from build123d import *

# Parameters (mm, degrees)
F0_W     = 12.5
F0_H     = 3
F0_W_2   = 6
F0_H_2   = 2
F0_W_3   = 44
F0_H_3   = 6
F0_H_4   = 1.2
F1_DEPTH = 580
F3_DEPTH = 50
F5_DEPTH = 50


with BuildPart() as f1:
    # F0 (on Right) → F1 (new body)
    with BuildSketch(Plane.YZ):
        with Locations((6.25, 1.5)):
            Rectangle(F0_W, F0_H)
        with Locations((15.5, 1.5)):
            Rectangle(F0_W_2, F0_H)
        with Locations((6.25, 4)):
            Rectangle(F0_W, F0_H_2)
        with Locations((40.5, 1.5)):
            Rectangle(F0_W_3, F0_H)
        with Locations((15.5, 4)):
            Rectangle(F0_W_2, F0_H_2)
        Polygon((18.5, 5), (18.5, 3), (62.5, 3), (52.9347826087, 5), align=None)
        with Locations((15.5, 8)):
            Rectangle(F0_W_2, F0_H_3)
        Polygon((18.5, 11), (18.5, 5), (52.9347826087, 5), (24.2391304348, 11), align=None)
        with Locations((15.5, 11.6)):
            Rectangle(F0_W_2, F0_H_4)
        Polygon((18.5, 12.2), (18.5, 11), (24.2391304348, 11), align=None)
    extrude(amount=F1_DEPTH)

    # F2 (on Top) → F3 (cut, symmetric)
    with BuildSketch(Plane.XY):
        Polygon((0, 62.5), (0, 0), (62.5, 0), align=None)
    extrude(amount=F3_DEPTH, both=True, mode=Mode.SUBTRACT)

    # F4 (on Top) → F5 (cut, symmetric)
    with BuildSketch(Plane.XY):
        Polygon((580, 62.5), (517.5, 0), (580, 0), align=None)
    extrude(amount=F5_DEPTH, both=True, mode=Mode.SUBTRACT)


solid = f1.part
Work out the finished part from the listing and answer in its coordinate system (mm). A direction names the side the tool comes from. Coordinates: 2 decimals unless noted, no trailing zeros. Order: outer loops, then holes, each group sorted by start corner. A loop starts at its lowest first (then second) coordinate and runs counter-clockwise, first axis right, second up. Notation, with made-up numbers: (-25, 6.25) - (22, 6.25) arc R22 cw to (22, 39.25) - close; hole circle Ø3 at (24, 73.25). An arc over 180 degrees is marked (long way). Put each result on its own line as item: value. Start each with the question number.
1) Find section B-B (y = 7). Give the vertices of the cut face in (x, z), plus the area to 4 significant figures.
2) Find section C-C (y = 45). Give the vertices of the cut face in (x, z).
3) Find the intervals of material crossed by line 1 (Z direction, x = 237, y = 6.5); line 2 (Z direction, x = 95, y = 39); line 3 (X direction, y = 38, z = 3.25), in increasing order. Write a range as from..to.
4) Flat-ended cylindrical pins translate along their axes: pin 1 (5 mm diameter, centred on y = 25.5, z = 8.5, fed in from -X); pin 2 (4 mm diameter, centred on x = 107, y = 54.5, fed in from +Z); pin 3 (10 mm diameter, centred on x = 272, y = 6.5, fed in from +Z). Find the tip coordinate at first contact, or state that the pin passes through.
5) For faces 4 (the flat face through (31.7, 30.8, 4.8)), 5 (the flat face through (287, 6, 5)), determine the directions among +Z, -Z, +X, -X, +Y, -Y from which every point of the face is accessible in a straight line to the end or side of a thin tool.
6) For a pull along Y with two mould halves and no side action, classify faces 1 (the flat face through (549.2, 31.7, 4.8)), 2 (the flat face through (286, 31, 0)), 3 (the flat face through (285.94, 40.808, 7.536)) as released by +Y, released by -Y, zero draft, split by the parting line, or undercut.
7) Find section A-A (x = 370). Give the vertices of the cut face in (y, z), plus the area to 3 significant figures.
Results list:
1. outline: (55.5, 0) - (524.5, 0) - (524.5, 5) - (55.5, 5) - close
1. area: 2,345 mm^2
2. outline: (17.5, 0) - (562.5, 0) - (562.5, 6.66) - (17.5, 6.66) - close
3. line 1: z = 0..5
3. line 2: z = 0..7.91
3. line 3: x = 24.5..555.5
4. pin 1: stops at x = 34.5
4. pin 2: stops at z = 5.09
4. pin 3: stops at z = 5
5. face 4: +Z, -Z, -X, -Y
5. face 5: +Z, +X, -X, -Y
6. face 1: released by -Y
6. face 2: zero draft
6. face 3: released by +Y
7. outline: (0, 0) - (62.5, 0) - (62.5, 3) - (18.5, 12.2) - (12.5, 12.2) - (12.5, 5) - (0, 5) - close
7. area: 470 mm^2
